from build123d import *

# Parameters (mm, degrees)
F0_W     = 47.7012
F0_H     = 31.8008
F0_R     = 2.1336
F1_DEPTH = 3.175
F2_DEPTH = 4.7752
F3_T     = -1.6002


with BuildPart() as f1:
    # F0 (on Top) → F1 (new body)
    with BuildSketch(Plane.XY):
        with Locations((-4.3733632303, 8.6500905454)):
            Rectangle(F0_W, F0_H)
        with Locations((-24.2615632303, -3.2625094546)):
            Circle(F0_R, mode=Mode.SUBTRACT)
        with Locations((-16.3113632303, -3.2625094546)):
            Circle(F0_R, mode=Mode.SUBTRACT)
        with Locations((-8.3611632303, -3.2625094546)):
            Circle(F0_R, mode=Mode.SUBTRACT)
        with Locations((-24.2615632303, 4.6876905454)):
            Circle(F0_R, mode=Mode.SUBTRACT)
        with Locations((-16.3113632303, 4.6876905454)):
            Circle(F0_R, mode=Mode.SUBTRACT)
        with Locations((-8.3611632303, 4.6876905454)):
            Circle(F0_R, mode=Mode.SUBTRACT)
        with Locations((-0.4109632303, -3.2625094546)):
            Circle(F0_R, mode=Mode.SUBTRACT)
        with Locations((7.5392367697, -3.2625094546)):
            Circle(F0_R, mode=Mode.SUBTRACT)
        with Locations((15.4894367697, -3.2625094546)):
            Circle(F0_R, mode=Mode.SUBTRACT)
        with Locations((-0.4109632303, 4.6876905454)):
            Circle(F0_R, mode=Mode.SUBTRACT)
        with Locations((7.5392367697, 4.6876905454)):
            Circle(F0_R, mode=Mode.SUBTRACT)
        with Locations((15.4894367697, 4.6876905454)):
            Circle(F0_R, mode=Mode.SUBTRACT)
        with Locations((-24.2615632303, 12.6378905454)):
            Circle(F0_R, mode=Mode.SUBTRACT)
        with Locations((-16.3113632303, 12.6378905454)):
            Circle(F0_R, mode=Mode.SUBTRACT)
        with Locations((-8.3611632303, 12.6378905454)):
            Circle(F0_R, mode=Mode.SUBTRACT)
        with Locations((-24.2615632303, 20.5880905454)):
            Circle(F0_R, mode=Mode.SUBTRACT)
        with Locations((-16.3113632303, 20.5880905454)):
            Circle(F0_R, mode=Mode.SUBTRACT)
        with Locations((-8.3611632303, 20.5880905454)):
            Circle(F0_R, mode=Mode.SUBTRACT)
        with Locations((-0.4109632303, 12.6378905454)):
            Circle(F0_R, mode=Mode.SUBTRACT)
        with Locations((7.5392367697, 12.6378905454)):
            Circle(F0_R, mode=Mode.SUBTRACT)
        with Locations((15.4894367697, 12.6378905454)):
            Circle(F0_R, mode=Mode.SUBTRACT)
        with Locations((-0.4109632303, 20.5880905454)):
            Circle(F0_R, mode=Mode.SUBTRACT)
        with Locations((7.5392367697, 20.5880905454)):
            Circle(F0_R, mode=Mode.SUBTRACT)
        with Locations((15.4894367697, 20.5880905454)):
            Circle(F0_R, mode=Mode.SUBTRACT)
    extrude(amount=F1_DEPTH)

    # F0 (on Top) → F2 (join)
    with BuildSketch(Plane.XY):
        with Locations((-24.2615632303, 20.5880905454)):
            Circle(F0_R)
        with Locations((-16.3113632303, 20.5880905454)):
            Circle(F0_R)
        with Locations((-8.3611632303, 20.5880905454)):
            Circle(F0_R)
        with Locations((-0.4109632303, 20.5880905454)):
            Circle(F0_R)
        with Locations((7.5392367697, 20.5880905454)):
            Circle(F0_R)
        with Locations((15.4894367697, 20.5880905454)):
            Circle(F0_R)
        with Locations((15.4894367697, 12.6378905454)):
            Circle(F0_R)
        with Locations((7.5392367697, 12.6378905454)):
            Circle(F0_R)
        with Locations((-0.4109632303, 12.6378905454)):
            Circle(F0_R)
        with Locations((-8.3611632303, 12.6378905454)):
            Circle(F0_R)
        with Locations((-16.3113632303, 12.6378905454)):
            Circle(F0_R)
        with Locations((-24.2615632303, 12.6378905454)):
            Circle(F0_R)
        with Locations((-24.2615632303, 4.6876905454)):
            Circle(F0_R)
        with Locations((-16.3113632303, 4.6876905454)):
            Circle(F0_R)
        with Locations((-8.3611632303, 4.6876905454)):
            Circle(F0_R)
        with Locations((-0.4109632303, 4.6876905454)):
            Circle(F0_R)
        with Locations((7.5392367697, 4.6876905454)):
            Circle(F0_R)
        with Locations((15.4894367697, 4.6876905454)):
            Circle(F0_R)
        with Locations((15.4894367697, -3.2625094546)):
            Circle(F0_R)
        with Locations((7.5392367697, -3.2625094546)):
            Circle(F0_R)
        with Locations((-0.4109632303, -3.2625094546)):
            Circle(F0_R)
        with Locations((-8.3611632303, -3.2625094546)):
            Circle(F0_R)
        with Locations((-16.3113632303, -3.2625094546)):
            Circle(F0_R)
        with Locations((-24.2615632303, -3.2625094546)):
            Circle(F0_R)
    extrude(amount=F2_DEPTH)

    # F3
    f3_openings = [f1.faces().sort_by_distance(p)[0] for p in [
        (-4.373363, 8.650091, 0),
    ]]
    offset(amount=F3_T, openings=f3_openings, kind=Kind.INTERSECTION)


solid = f1.part
Geometry check sheet. Reference: the model listing, model coordinates, mm. A direction names the side the tool comes from. Give positions to 0.01 mm unless a question says otherwise; leave off trailing zeros. Order: outer loops, then holes, each group sorted by start corner. A loop starts at its lowest first (then second) coordinate and runs counter-clockwise, first axis right, second up.
1. Sectioned sample at C-C (x = 12.5). Record the boundary of the cut face in (y, z) (1 decimal), then the cut area to 3 significant figures.
Completed:
outline: (-7.3, 0) - (-5.7, 0) - (-5.7, 1.6) - (23, 1.6) - (23, 0) - (24.6, 0) - (24.6, 3.2) - (-7.3, 3.2) - close
area: 55.9 mm2
2. Scan lines: line 1 (Y direction, x = -7, z = 0.8); line 2 (X direction, y = 8, z = 1.05); line 3 (Y direction, x = -6.5, z = 4.1). Record each from-to range of solid material in increasing order.
Completed:
line 1: y = -7.25 to -5.65, 22.95 to 24.55
line 2: x = -28.22 to -26.62, 17.88 to 19.48
line 3: y = -4.31 to -2.22, 3.64 to 5.73, 11.59 to 13.68, 19.54 to 21.63
3. Depth check by flat-ended pin: pin 1 (1.2 mm diameter, centred on x = 7.54, y = -3.26, fed in from -Z); pin 2 (0.5 mm diameter, centred on x = 15.5, y = 20.5, fed in from -Z) (3 decimals). Enter the tip coordinate at first touch or a pass-through.
Completed:
pin 1: stops at z = 1.57
pin 2: stops at z = 3.175
4. Sectioned sample at D-D (z = 3.75). State how many separate pieces and enclosed holes the cut face has, then the cut area to 3 significant figures.
Completed:
separate pieces: 24
enclosed holes: 0
area: 343 mm2
5. Access from +Z, -Z, +X, -X, +Y, -Y to the whole of each face (thin tool, end or side, straight path). Record for faces 4 (the face through (8.686, 6.487, 3.964)), 5 (the face through (-16, 5, 4.775)), 6 (the face through (-0.165, 12.165, 2.364)).
Completed:
face 4: +Z
face 5: +Z, +X, -X, +Y, -Y
face 6: -Z
6. Sectioned sample at A-A (z = 1.05). Record the boundary of the cut face in (x, y), then the cut area to 3 significant figures.
Completed:
outline: (-28.22, -7.25) - (19.48, -7.25) - (19.48, 24.55) - (-28.22, 24.55) - close; hole (-26.62, -5.65) - (17.88, -5.65) - (17.88, 22.95) - (-26.62, 22.95) - close
area: 244 mm2
7. Draft check along X on faces 1 (the face through (-7.377, 10.745, 3.964)), 2 (the face through (-24, 5, 4.775)), 3 (the face through (-16.705, 20.949, 2.364)). Enter one of: pulls with the +X half, pulls with the -X half, needs draft (parallel to the pull), parting line crosses it, or undercut.
Completed:
face 1: undercut
face 2: needs draft
face 3: undercut
8. Sectioned sample at B-B (y = 2). Record the boundary of the cut face in (x, z) (3 decimals), then the cut area to 3 significant figures.
Completed:
outline: (-28.224, 0) - (-26.624, 0) - (-26.624, 1.575) - (17.877, 1.575) - (17.877, 0) - (19.477, 0) - (19.477, 3.175) - (-28.224, 3.175) - close
area: 81.4 mm2
